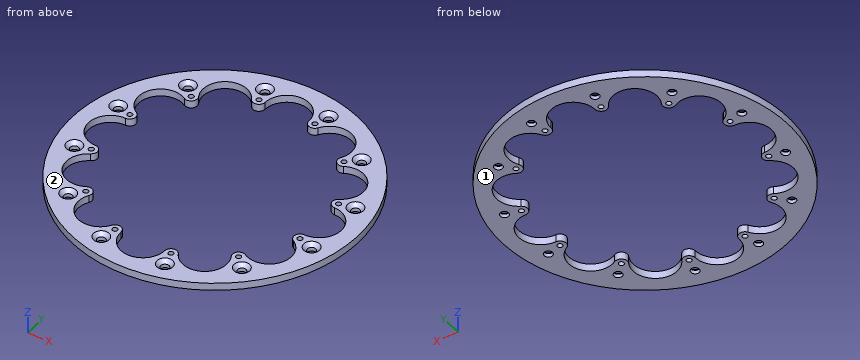
```python
from build123d import *

# Parameters (mm, degrees)
EXTRUDE_1_OUTLINE_R      = 58.25
EXTRUDE_1_OUTLINE_R_2    = 1.55
EXTRUDE_1_OUTLINE_R_3    = 1.05
EXTRUDE_1_OUTLINE_R_4    = 1.549999992
EXTRUDE_1_OUTLINE_R_5    = 1.550000008
EXTRUDE_1_DEPTH          = 3
PATTERN_CIRCULAR_1_COUNT = 12


# Read off the part's stored shape, not the designer's step: 凸台-拉伸1
with BuildPart() as part:
    # 凸台-拉伸1 outline → 凸台-拉伸1 (new body)
    with BuildSketch(Plane.XY):
        Circle(EXTRUDE_1_OUTLINE_R)
        with Locations((-35.710722211, -35.710722211)):
            Circle(EXTRUDE_1_OUTLINE_R_2, mode=Mode.SUBTRACT)
        with Locations((-31.418584049, -31.418584049)):
            Circle(EXTRUDE_1_OUTLINE_R_3, mode=Mode.SUBTRACT)
        with Locations((-13.071031517, -48.781753727)):
            Circle(EXTRUDE_1_OUTLINE_R_2, mode=Mode.SUBTRACT)
        with Locations((-11.499999913, -42.918583962)):
            Circle(EXTRUDE_1_OUTLINE_R_3, mode=Mode.SUBTRACT)
        with Locations((-48.781753727, -13.071031517)):
            Circle(EXTRUDE_1_OUTLINE_R_2, mode=Mode.SUBTRACT)
        with Locations((-42.918583962, -11.499999913)):
            Circle(EXTRUDE_1_OUTLINE_R_3, mode=Mode.SUBTRACT)
        with Locations((13.071031517, -48.781753727)):
            Circle(EXTRUDE_1_OUTLINE_R_4, mode=Mode.SUBTRACT)
        with Locations((11.499999913, -42.918583962)):
            Circle(EXTRUDE_1_OUTLINE_R_3, mode=Mode.SUBTRACT)
        with Locations((35.710722211, -35.710722211)):
            Circle(EXTRUDE_1_OUTLINE_R_2, mode=Mode.SUBTRACT)
        with Locations((31.418584049, -31.418584049)):
            Circle(EXTRUDE_1_OUTLINE_R_3, mode=Mode.SUBTRACT)
        with Locations((42.918583962, -11.499999913)):
            Circle(EXTRUDE_1_OUTLINE_R_3, mode=Mode.SUBTRACT)
        with Locations((48.781753727, -13.071031517)):
            Circle(EXTRUDE_1_OUTLINE_R_2, mode=Mode.SUBTRACT)
        with Locations((-48.781753727, 13.071031517)):
            Circle(EXTRUDE_1_OUTLINE_R_2, mode=Mode.SUBTRACT)
        with Locations((-42.918583962, 11.499999913)):
            Circle(EXTRUDE_1_OUTLINE_R_3, mode=Mode.SUBTRACT)
        with Locations((-31.418584049, 31.418584049)):
            Circle(EXTRUDE_1_OUTLINE_R_3, mode=Mode.SUBTRACT)
        with Locations((-35.710722211, 35.710722211)):
            Circle(EXTRUDE_1_OUTLINE_R_2, mode=Mode.SUBTRACT)
        with Locations((-11.499999913, 42.918583962)):
            Circle(EXTRUDE_1_OUTLINE_R_3, mode=Mode.SUBTRACT)
        with Locations((-13.071031517, 48.781753727)):
            Circle(EXTRUDE_1_OUTLINE_R_5, mode=Mode.SUBTRACT)
        with BuildLine():
            ThreePointArc((-42.918891796, 8.999999932), (-40.503769396, 10.8529523), (-41.668850564, 13.665217323))
            ThreePointArc((-41.668850564, 13.665217323), (-44.964038964, 25.96), (-32.668850632, 29.253674473))
            ThreePointArc((-32.668850632, 29.253674473), (-29.650817096, 29.650817096), (-29.253674473, 32.668850632))
            ThreePointArc((-29.253674473, 32.668850632), (-25.96, 44.964038964), (-13.665217323, 41.668850564))
            ThreePointArc((-13.665217323, 41.668850564), (-10.852952298, 40.503769388), (-8.999999924, 42.918891796))
            ThreePointArc((-8.999999924, 42.918891796), (0, 51.92), (8.999999932, 42.918891796))
            ThreePointArc((8.999999932, 42.918891796), (10.8529523, 40.503769396), (13.665217323, 41.668850564))
            ThreePointArc((13.665217323, 41.668850564), (25.96, 44.964038964), (29.253674473, 32.668850632))
            ThreePointArc((29.253674473, 32.668850632), (29.650817096, 29.650817096), (32.668850632, 29.253674473))
            ThreePointArc((32.668850632, 29.253674473), (44.964038964, 25.96), (41.668850564, 13.665217323))
            ThreePointArc((41.668850564, 13.665217323), (40.503769396, 10.8529523), (42.918891796, 8.999999932))
            ThreePointArc((42.918891796, 8.999999932), (51.92, 0), (42.918891796, -8.999999932))
            ThreePointArc((42.918891796, -8.999999932), (40.503769396, -10.8529523), (41.668850564, -13.665217323))
            ThreePointArc((41.668850564, -13.665217323), (44.964038964, -25.96), (32.668850632, -29.253674473))
            ThreePointArc((32.668850632, -29.253674473), (29.650817096, -29.650817096), (29.253674473, -32.668850632))
            ThreePointArc((29.253674473, -32.668850632), (25.96, -44.964038964), (13.665217323, -41.668850564))
            ThreePointArc((13.665217323, -41.668850564), (10.852952302, -40.503769404), (8.99999994, -42.918891796))
            ThreePointArc((8.99999994, -42.918891796), (0, -51.92), (-8.999999932, -42.918891796))
            ThreePointArc((-8.999999932, -42.918891796), (-10.8529523, -40.503769396), (-13.665217323, -41.668850564))
            ThreePointArc((-13.665217323, -41.668850564), (-25.96, -44.964038964), (-29.253674473, -32.668850632))
            ThreePointArc((-29.253674473, -32.668850632), (-29.650817096, -29.650817096), (-32.668850632, -29.253674473))
            ThreePointArc((-32.668850632, -29.253674473), (-44.964038964, -25.96), (-41.668850564, -13.665217323))
            ThreePointArc((-41.668850564, -13.665217323), (-40.503769396, -10.8529523), (-42.918891796, -8.999999932))
            ThreePointArc((-42.918891796, -8.999999932), (-51.92, 0), (-42.918891796, 8.999999932))
        make_face(mode=Mode.SUBTRACT)
        with Locations((42.918583962, 11.499999913)):
            Circle(EXTRUDE_1_OUTLINE_R_3, mode=Mode.SUBTRACT)
        with Locations((48.781753727, 13.071031517)):
            Circle(EXTRUDE_1_OUTLINE_R_2, mode=Mode.SUBTRACT)
        with Locations((11.499999913, 42.918583962)):
            Circle(EXTRUDE_1_OUTLINE_R_3, mode=Mode.SUBTRACT)
        with Locations((13.071031517, 48.781753727)):
            Circle(EXTRUDE_1_OUTLINE_R_2, mode=Mode.SUBTRACT)
        with Locations((31.418584049, 31.418584049)):
            Circle(EXTRUDE_1_OUTLINE_R_3, mode=Mode.SUBTRACT)
        with Locations((35.710722211, 35.710722211)):
            Circle(EXTRUDE_1_OUTLINE_R_2, mode=Mode.SUBTRACT)
    extrude(amount=EXTRUDE_1_DEPTH)

    # 草图4 → M3 开槽半沉头螺钉的锥形沉头孔1 (revolve, cut)
    with BuildSketch(Plane(origin=(-13.071031517, 48.781753727, 3), x_dir=(0, -1, 0), z_dir=(1, 0, 0))):
        Polygon((0, 0), (0, 21.021463052), (1.7, 20), (1.7, 1.5), (3.2, 0), align=None)
    hole_wizard_m3_1 = revolve(axis=Axis((-13.071031517, 48.781753727, 9.35), (0, 0, -1)), mode=Mode.SUBTRACT)

    # 阵列(圆周)1: M3 开槽半沉头螺钉的锥形沉头孔1 ×12 about axis
    pattern_circular_1_axis = Axis((0, 0, 0), (0, 0, 1))
    for i in range(1, PATTERN_CIRCULAR_1_COUNT):
        add(hole_wizard_m3_1.rotate(pattern_circular_1_axis, i * 360 / PATTERN_CIRCULAR_1_COUNT), mode=Mode.SUBTRACT)


solid = part.part
```
Source: CAD feature listing. Evaluate the final solid. Frame: model axes, mm. Face numbers are marked on the shaded views. Round coordinates to 2 decimals unless told otherwise and drop trailing zeros. Order: outer loops, then holes, each group sorted by start corner. A loop starts at its lowest first (then second) coordinate and runs counter-clockwise, first axis right, second up. Notation, with made-up numbers: (-13, 15.5) -> (-5, 15.5) arc R9 ccw to (-5, 27.5) -> close; hole circle Ø11 at (25, 58). An arc over 180 degrees is marked (long way). One line per item, written item: value. Start each with the question number.
Q1. Section query B-B (y = 25.5). Return the cut outline in (x, z).
Q2. Section query A-A (x = -1). Return the cut outline in (y, z), plus the area to 3 significant figures.
Q3. Section query C-C (z = 2.45). Give the number of separate pieces and of enclosed holes in the cut face, plus the area to 3 significant figures.
Q4. Draft query along Z for the marked faces 1 and 2. Return one class per face: pulls with the +Z half, pulls with the -Z half, needs draft (parallel to the pull), parting line crosses it, or undercut.
Q5. Pin query (flat end, axial travel): pin 1 (3 mm diameter, centred on x = -13.07, y = 48.78, fed in from +Z) (1 decimal); pin 2 (4 mm diameter, centred on x = -13.07, y = -48.78, fed in from +Z); pin 3 (1 mm diameter, centred on y = 40.5, z = 2, fed in from -X). Return the tip coordinate at first contact, or that it passes through.
Q6. Material intervals for probe 1 along Y at (x, z) = (12, 0.2); probe 2 along X at (y, z) = (-34.5, 0.45); probe 3 along Y at (x, z) = (0, 1.4), sorted ascending.
Findings below:
1. outline: (-52.37, 0) -> (-45.21, 0) -> (-45.21, 3) -> (-52.37, 3) -> close; (45.21, 0) -> (52.37, 0) -> (52.37, 3) -> (45.21, 3) -> close
2. outline: (-58.24, 0) -> (-51.86, 0) -> (-51.86, 3) -> (-58.24, 3) -> close; (51.86, 0) -> (58.24, 0) -> (58.24, 3) -> (51.86, 3) -> close
2. area: 38.3 mm²
3. separate pieces: 1
3. enclosed holes: 25
3. area: 3,000 mm²
4. face 1: pulls with the -Z half
4. face 2: pulls with the +Z half
5. pin 1: through
5. pin 2: z = 1.8
5. pin 3: x = -42.34
6. probe 1: -57 to -50.1, -47.46 to -43.84, -42 to -40.47, 40.47 to 42, 43.84 to 47.46, 50.1 to 57
6. probe 2: -46.93 to -36.9, -34.52 to -30.05, 30.05 to 34.52, 36.9 to 46.93
6. probe 3: -58.25 to -51.92, 51.92 to 58.25
